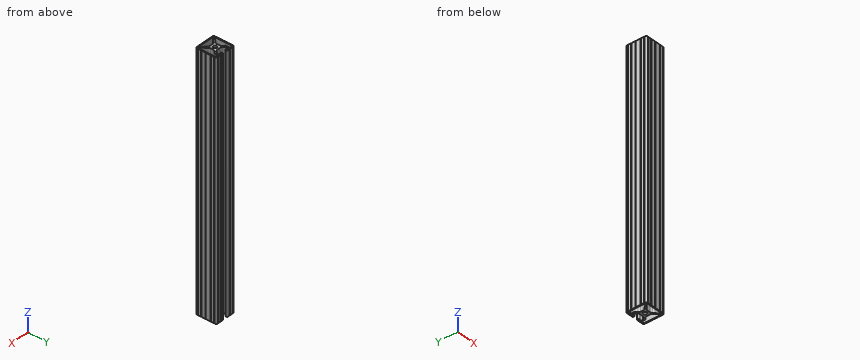
```python
from build123d import *

# Parameters (mm, degrees)
SKETCH1_R      = 3.3274
EXTRUDE1_DEPTH = 457.2


with BuildPart() as part:
    # Sketch1 → Extrude1 (new body)
    with BuildSketch(Plane.XY):
        with BuildLine():
            Line((6.814144258, 15.824710921), (9.017, 15.824710921))
            ThreePointArc((9.017, 15.824710921), (9.915025612, 15.452736533), (10.287, 14.554710921))
            Line((10.287, 14.554710921), (10.287, 12.815421755))
            ThreePointArc((10.287, 12.815421755), (10.219314574, 12.47518159), (10.026564972, 12.186750874))
            Line((10.026564972, 12.186750874), (6.100754025, 8.261601293))
            ThreePointArc((6.100754025, 8.261601293), (4.55990611, 7.23218044), (2.742421178, 6.8707))
            Line((2.742421178, 6.8707), (-2.742421178, 6.8707))
            ThreePointArc((-2.742421178, 6.8707), (-4.55990611, 7.23218044), (-6.100754025, 8.261601293))
            Line((-6.100754025, 8.261601293), (-10.026564972, 12.186750874))
            ThreePointArc((-10.026564972, 12.186750874), (-10.219314574, 12.47518159), (-10.287, 12.815421755))
            Line((-10.287, 12.815421755), (-10.287, 14.554710921))
            ThreePointArc((-10.287, 14.554710921), (-9.915025612, 15.452736533), (-9.017, 15.824710921))
            Line((-9.017, 15.824710921), (-6.814144258, 15.824710921))
            Line((-6.814144258, 15.824710921), (-6.814144258, 14.986))
            Line((-6.814144258, 14.986), (-5.6388, 14.986))
            ThreePointArc((-5.6388, 14.986), (-4.525248241, 15.447248241), (-4.064, 16.5608))
            Line((-4.064, 16.5608), (-4.064, 17.4752))
            ThreePointArc((-4.064, 17.4752), (-4.525248241, 18.588751759), (-5.6388, 19.05))
            Line((-5.6388, 19.05), (-7.9756, 19.05))
            ThreePointArc((-7.9756, 19.05), (-8.7376, 18.288), (-9.4996, 19.05))
            Line((-9.4996, 19.05), (-14.3256, 19.05))
            ThreePointArc((-14.3256, 19.05), (-15.0876, 18.288), (-15.8496, 19.05))
            Line((-15.8496, 19.05), (-15.875, 19.05))
            ThreePointArc((-15.875, 19.05), (-18.12006403, 18.12006403), (-19.05, 15.875))
            Line((-19.05, 15.875), (-19.05, 15.8496))
            ThreePointArc((-19.05, 15.8496), (-18.288, 15.0876), (-19.05, 14.3256))
            Line((-19.05, 14.3256), (-19.05, 9.4996))
            ThreePointArc((-19.05, 9.4996), (-18.288, 8.7376), (-19.05, 7.9756))
            Line((-19.05, 7.9756), (-19.05, 0.762))
            ThreePointArc((-19.05, 0.762), (-18.288, 0), (-19.05, -0.762))
            Line((-19.05, -0.762), (-19.05, -7.9756))
            ThreePointArc((-19.05, -7.9756), (-18.288, -8.7376), (-19.05, -9.4996))
            Line((-19.05, -9.4996), (-19.05, -14.3256))
            ThreePointArc((-19.05, -14.3256), (-18.288, -15.0876), (-19.05, -15.8496))
            Line((-19.05, -15.8496), (-19.05, -15.875))
            ThreePointArc((-19.05, -15.875), (-18.12006403, -18.12006403), (-15.875, -19.05))
            Line((-15.875, -19.05), (-15.8496, -19.05))
            ThreePointArc((-15.8496, -19.05), (-15.0876, -18.288), (-14.3256, -19.05))
            Line((-14.3256, -19.05), (-9.4996, -19.05))
            ThreePointArc((-9.4996, -19.05), (-8.7376, -18.288), (-7.9756, -19.05))
            Line((-7.9756, -19.05), (-0.762, -19.05))
            ThreePointArc((-0.762, -19.05), (0, -18.288), (0.762, -19.05))
            Line((0.762, -19.05), (7.9756, -19.05))
            ThreePointArc((7.9756, -19.05), (8.7376, -18.288), (9.4996, -19.05))
            Line((9.4996, -19.05), (14.3256, -19.05))
            ThreePointArc((14.3256, -19.05), (15.0876, -18.288), (15.8496, -19.05))
            Line((15.8496, -19.05), (15.875, -19.05))
            ThreePointArc((15.875, -19.05), (18.12006403, -18.12006403), (19.05, -15.875))
            Line((19.05, -15.875), (19.05, -15.8496))
            ThreePointArc((19.05, -15.8496), (18.288, -15.0876), (19.05, -14.3256))
            Line((19.05, -14.3256), (19.05, -9.4996))
            ThreePointArc((19.05, -9.4996), (18.288, -8.7376), (19.05, -7.9756))
            Line((19.05, -7.9756), (19.05, -0.762))
            ThreePointArc((19.05, -0.762), (18.288, 0), (19.05, 0.762))
            Line((19.05, 0.762), (19.05, 7.9756))
            ThreePointArc((19.05, 7.9756), (18.288, 8.7376), (19.05, 9.4996))
            Line((19.05, 9.4996), (19.05, 14.3256))
            ThreePointArc((19.05, 14.3256), (18.288, 15.0876), (19.05, 15.8496))
            Line((19.05, 15.8496), (19.05, 15.875))
            ThreePointArc((19.05, 15.875), (18.12006403, 18.12006403), (15.875, 19.05))
            Line((15.875, 19.05), (15.8496, 19.05))
            ThreePointArc((15.8496, 19.05), (15.0876, 18.288), (14.3256, 19.05))
            Line((14.3256, 19.05), (9.4996, 19.05))
            ThreePointArc((9.4996, 19.05), (8.7376, 18.288), (7.9756, 19.05))
            Line((7.9756, 19.05), (5.6388, 19.05))
            ThreePointArc((5.6388, 19.05), (4.525248241, 18.588751759), (4.064, 17.4752))
            Line((4.064, 17.4752), (4.064, 16.5608))
            ThreePointArc((4.064, 16.5608), (4.525248241, 15.447248241), (5.6388, 14.986))
            Line((5.6388, 14.986), (6.814144258, 14.986))
            Line((6.814144258, 14.986), (6.814144258, 15.824710921))
        make_face()
        Circle(SKETCH1_R, mode=Mode.SUBTRACT)
        with BuildLine():
            Line((17.272, -15.193619561), (17.272, 14.478))
            ThreePointArc((17.272, 14.478), (16.453656347, 16.453656347), (14.478, 17.272))
            Line((14.478, 17.272), (12.554627238, 17.272))
            ThreePointArc((12.554627238, 17.272), (12.285219554, 17.160407684), (12.173627238, 16.891))
            Line((12.173627238, 16.891), (12.173627238, 11.224276306))
            ThreePointArc((12.173627238, 11.224276306), (11.931893574, 10.009132858), (11.243502135, 8.979023159))
            Line((11.243502135, 8.979023159), (8.147867153, 5.883909687))
            ThreePointArc((8.147867153, 5.883909687), (7.118033561, 4.342865578), (6.7564, 2.525010979))
            Line((6.7564, 2.525010979), (6.7564, -2.638829998))
            ThreePointArc((6.7564, -2.638829998), (7.117934192, -4.456444709), (8.147499936, -5.99736151))
            Line((8.147499936, -5.99736151), (10.978133922, -8.828137555))
            ThreePointArc((10.978133922, -8.828137555), (11.047042355, -8.907266312), (11.104427332, -8.995111041))
            Line((11.104427332, -8.995111041), (12.13998256, -10.847500325))
            ThreePointArc((12.13998256, -10.847500325), (12.197373304, -10.935352679), (12.266289489, -11.014487331))
            Line((12.266289489, -11.014487331), (16.687520892, -15.435718734))
            ThreePointArc((16.687520892, -15.435718734), (17.060643194, -15.509937374), (17.272, -15.193619561))
        make_face(mode=Mode.SUBTRACT)
        with BuildLine():
            Line((-12.173627238, 11.224276306), (-12.173627238, 16.891))
            ThreePointArc((-12.173627238, 16.891), (-12.285219554, 17.160407684), (-12.554627238, 17.272))
            Line((-12.554627238, 17.272), (-14.478, 17.272))
            ThreePointArc((-14.478, 17.272), (-16.453656347, 16.453656347), (-17.272, 14.478))
            Line((-17.272, 14.478), (-17.272, -15.193619561))
            ThreePointArc((-17.272, -15.193619561), (-17.060643194, -15.509937374), (-16.687520892, -15.435718734))
            Line((-16.687520892, -15.435718734), (-12.266289488, -11.014487333))
            ThreePointArc((-12.266289488, -11.014487333), (-12.197373302, -10.935352681), (-12.139982558, -10.847500326))
            Line((-12.139982558, -10.847500326), (-11.104427331, -8.995111042))
            ThreePointArc((-11.104427331, -8.995111042), (-11.047042353, -8.907266313), (-10.978133921, -8.828137556))
            Line((-10.978133921, -8.828137556), (-8.147499934, -5.997361511))
            ThreePointArc((-8.147499934, -5.997361511), (-7.11793419, -4.45644471), (-6.756399998, -2.638829999))
            Line((-6.756399998, -2.638829999), (-6.756399998, 2.525010979))
            ThreePointArc((-6.756399998, 2.525010979), (-7.118033559, 4.342865578), (-8.147867152, 5.883909688))
            Line((-8.147867152, 5.883909688), (-11.243502135, 8.979023158))
            ThreePointArc((-11.243502135, 8.979023158), (-11.931893574, 10.009132857), (-12.173627238, 11.224276306))
        make_face(mode=Mode.SUBTRACT)
        with BuildLine():
            Line((15.358897182, -16.621566737), (11.090984974, -12.353654529))
            ThreePointArc((11.090984974, -12.353654529), (11.011857946, -12.284744111), (10.924014656, -12.227356929))
            Line((10.924014656, -12.227356929), (9.072208991, -11.192066981))
            ThreePointArc((9.072208991, -11.192066981), (8.984358076, -11.134674031), (8.905225153, -11.06575586))
            Line((8.905225153, -11.06575586), (6.101578488, -8.261968492))
            ThreePointArc((6.101578488, -8.261968492), (4.560603247, -7.232279806), (2.742878424, -6.870700004))
            Line((2.742878424, -6.870700004), (-2.742878422, -6.870700004))
            ThreePointArc((-2.742878422, -6.870700004), (-4.560603245, -7.232279806), (-6.101578486, -8.261968491))
            Line((-6.101578486, -8.261968491), (-8.905225151, -11.06575586))
            ThreePointArc((-8.905225151, -11.06575586), (-8.984358074, -11.134674031), (-9.072208989, -11.19206698))
            Line((-9.072208989, -11.19206698), (-10.924014654, -12.227356929))
            ThreePointArc((-10.924014654, -12.227356929), (-11.011857944, -12.284744111), (-11.090984971, -12.353654529))
            Line((-11.090984971, -12.353654529), (-15.35889718, -16.621566737))
            ThreePointArc((-15.35889718, -16.621566737), (-15.441490846, -17.036793139), (-15.0894789, -17.272000001))
            Line((-15.0894789, -17.272000001), (15.089478903, -17.272000001))
            ThreePointArc((15.089478903, -17.272000001), (15.441490849, -17.036793139), (15.358897182, -16.621566737))
        make_face(mode=Mode.SUBTRACT)
    extrude(amount=-EXTRUDE1_DEPTH)


solid = part.part
```
Check sheet for the modelled part. Datum: model origin and axes. Units: mm. Round coordinates to 2 decimals unless told otherwise and drop trailing zeros.
1) Section check A-A (z = -313). Give the number of separate pieces and of enclosed holes in the cut face, and give its area (3 significant figures).
2) Scan lines: line 1 (X direction, y = 6, z = -393); line 2 (Y direction, x = 0, z = -269.5); line 3 (Y direction, x = 9, z = -367). Record each from-to range of solid material in increasing order.
3) Go/stop test with flat-tipped pins: pin 1 Ø8 at (x, y) = (-4, -12) entering from -Z; pin 2 Ø0.5 at (y, z) = (17, -134) entering from -X; pin 3 Ø2.5 at (x, z) = (0.5, -282.5) entering from +Y. Record where each tip stops, or that it passes through.
Result:
1. separate pieces: 1
1. enclosed holes: 4
1. area: 534 mm2
2. line 1: x = -19.05 to -17.27, -8.26 to 8.26, 17.27 to 19.05
2. line 2: y = -18.29 to -17.27, -6.87 to -3.33, 3.33 to 6.87
2. line 3: y = -18.33 to -17.27, -11.15 to -6.85, 6.74 to 11.16, 15.82 to 18.33
3. pin 1: passes through
3. pin 2: stops at x = -18.93
3. pin 3: stops at y = 6.87
